Autodesk Inventor part; units mm, degrees
ref_plane "YZ Plane" through (0, 0, 0) normal (1, 0, 0) x (0, 1, 0)
ref_plane "XZ Plane" through (0, 0, 0) normal (0, 1, 0) x (-1, 0, 0)
ref_plane "XY Plane" through (0, 0, 0) normal (0, 0, 1) x (1, 0, 0)
sketch "Sketch1" plane through (0, 0, 0) normal (0, 1, 0) x (-1, 0, 0)
  line L0 (-43.6562, 8.7312) -> (-43.6562, -8.7312)
  line L1 (-43.6562, -8.7312) -> (43.6562, -8.7312)
  line L2 (43.6562, -8.7312) -> (43.6562, 8.7312)
  line L3 (43.6562, 8.7312) -> (-43.6562, 8.7312)
  line L4 (-43.6562, 8.7312) -> (43.6562, -8.7312) construction
  line L5 (-43.6562, -8.7312) -> (43.6562, 8.7312) construction
  line L6 (-40.4812, 5.5563) -> (-40.4812, -5.5563)
  line L7 (-40.4812, -5.5563) -> (40.4812, -5.5563)
  line L8 (40.4812, -5.5563) -> (40.4812, 5.5563)
  line L9 (40.4812, 5.5563) -> (-40.4812, 5.5563)
  line L10 (-40.4812, 5.5563) -> (40.4812, -5.5563) construction
  line L11 (-40.4812, -5.5563) -> (40.4812, 5.5563) construction
  point P0 (0, 0)
  dimension "d0" = 17.4625
  dimension "d1" = 87.3125
  dimension "d2" = 3.175
  dimension "d3" = 3.175
extrude "Extrusion1" add sketch "Sketch1" along normal blind 50.8
properties part number "spacer-0_6875x3_4375"
Geometry check sheet. Reference: the model listing, model coordinates, mm. A direction names the side the tool comes from. Coordinates: 2 decimals unless noted, no trailing zeros. Order: outer loops, then holes, each group sorted by start corner. A loop starts at its lowest first (then second) coordinate and runs counter-clockwise, first axis right, second up.
Item 1: Scan lines: line 1 along Z through (x, y) = (-29, 32.5); line 2 along X through (y, z) = (30, -5). Record each from-to range of solid material in increasing order.
Item 2: Mould release check, pull along X, two halves, no side actions. Record for faces 1 (the flat face through (-43.656, 25, 0)), 2 (the flat face through (43.656, 25, 0)), 3 (the flat face through (40.481, 25, 0)): released by +X, released by -X, zero draft, split by the parting line, or undercut.
Item 3: Section check A-A (y = 38.5). Enter the section's corners in (x, z).
Item 4: Section check B-B (z = 4.5). Enter the section's corners in (x, y).
Item 5: Tool access check on faces 4 (the flat face through (-1, 25, 5.556)), 5 (the flat face through (-1, 25, 8.731)). Record the directions out of +Z, -Z, +X, -X, +Y, -Y that give a thin tool (end or side, any length) a straight path to the whole face; none if there is none.
Item 6: Section check C-C (x = 34.5). Enter the section's corners in (y, z).
Check sheet entries:
1. line 1: z = -8.73 to -5.56, 5.56 to 8.73
1. line 2: x = -43.66 to -40.48, 40.48 to 43.66
2. face 1: released by -X
2. face 2: released by +X
2. face 3: undercut
3. outline: (-43.66, -8.73) - (43.66, -8.73) - (43.66, 8.73) - (-43.66, 8.73) - close; hole (-40.48, -5.56) - (40.48, -5.56) - (40.48, 5.56) - (-40.48, 5.56) - close
4. outline: (-43.66, 0) - (-40.48, 0) - (-40.48, 50.8) - (-43.66, 50.8) - close; (40.48, 0) - (43.66, 0) - (43.66, 50.8) - (40.48, 50.8) - close
5. face 4: +Y, -Y
5. face 5: +Z, +X, -X, +Y, -Y
6. outline: (0, -8.73) - (50.8, -8.73) - (50.8, -5.56) - (0, -5.56) - close; (0, 5.56) - (50.8, 5.56) - (50.8, 8.73) - (0, 8.73) - close
